Part model, mm, in its own coordinate system. Face numbers are marked on the shaded views. A direction names the side the tool comes from. Give positions to 0.01 mm unless a question says otherwise; leave off trailing zeros. Order: outer loops, then holes, each group sorted by start corner. A loop starts at its lowest first (then second) coordinate and runs counter-clockwise, first axis right, second up. Notation, with made-up numbers: M 65,37.25 L 111,37.25 A14 cw 111,62.25 Z; hole C 56,-14 d8. An arc over 180 degrees is marked long. One line per question, with ' | ' between items.
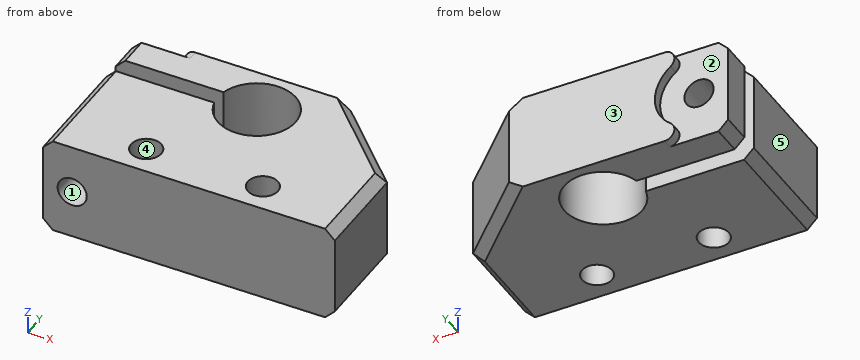
```python
from build123d import *

# Parameters (mm, degrees)
SKETCH3_W                    = 30
SKETCH3_H                    = 8
SKETCH3_R                    = 1.55
BOSS_EXTRUDE1_DEPTH          = 5
SKETCH6_R                    = 4
BOSS_EXTRUDE2_DEPTH          = 10
SKETCH8_W                    = 15
SKETCH8_H                    = 1.8
CUT_EXTRUDE_THIN1_DEPTH      = 1
CUT_EXTRUDE_THIN1_DEPTH_BACK = 11
SKETCH9_R                    = 1.5
CUT_EXTRUDE1_DEPTH           = 19
CUT_EXTRUDE2_DEPTH           = 1
CHAMFER2_SIZE                = 1


with BuildPart() as part:
    # Sketch3 → Boss-Extrude1 (new body, symmetric)
    with BuildSketch(Plane.XY):
        Rectangle(SKETCH3_W, SKETCH3_H)
        with Locations((-6, -1)):
            Circle(SKETCH3_R, mode=Mode.SUBTRACT)
        with Locations((6, -1)):
            Circle(SKETCH3_R, mode=Mode.SUBTRACT)
    extrude(amount=BOSS_EXTRUDE1_DEPTH, both=True)

    # Sketch6 → Boss-Extrude2 (add)
    with BuildSketch(Plane.XY.offset(5)):
        Polygon((-15, 4), (15, 4), (15, 6), (7, 14), (-15, 14), align=None)
        with Locations((0, 9)):
            Circle(SKETCH6_R, mode=Mode.SUBTRACT)
    extrude(amount=-BOSS_EXTRUDE2_DEPTH)

    # Sketch8 → Cut-Extrude-Thin1 (cut, two sides)
    with BuildSketch(Plane.XY.offset(5)) as cut_extrude_thin1_sk:
        with Locations((-7.5, 9)):
            Rectangle(SKETCH8_W, SKETCH8_H)
    extrude(amount=CUT_EXTRUDE_THIN1_DEPTH, mode=Mode.SUBTRACT)
    extrude(cut_extrude_thin1_sk.sketch, amount=-CUT_EXTRUDE_THIN1_DEPTH_BACK, mode=Mode.SUBTRACT)

    # Sketch9 → Cut-Extrude1 (cut, through all)
    with BuildSketch(Plane(origin=(0, 14, 0), x_dir=(1, 0, 0), z_dir=(0, 1, 0))):
        with Locations((-12, 0)):
            Circle(SKETCH9_R)
    extrude(amount=-CUT_EXTRUDE1_DEPTH, mode=Mode.SUBTRACT)

    # Sketch10 → Cut-Extrude2 (cut)
    with BuildSketch(Plane(origin=(0, 14, 0), x_dir=(1, 0, 0), z_dir=(0, 1, 0))):
        with BuildLine():
            Line((-9, 5), (-15, 5))
            Line((-15, 5), (-15, -5))
            Line((-15, -5), (-9, -5))
            ThreePointArc((-9, -5), (-9.948683298, -4.316227766), (-9.6, -3.2))
            ThreePointArc((-9.6, -3.2), (-8, 0), (-9.6, 3.2))
            ThreePointArc((-9.6, 3.2), (-9.948683298, 4.316227766), (-9, 5))
        make_face()
    extrude(amount=-CUT_EXTRUDE2_DEPTH, mode=Mode.SUBTRACT)

    # Chamfer2
    chamfer2_edges = [part.edges().sort_by_distance(p)[0] for p in [
        (11, 10, -5),
        (11, 10, 5),
        (-15, 2.05, -5),
        (-15, 2.05, 5),
        (15, 1, 5),
        (15, 1, -5),
        (-15, 11.45, -5),
        (-15, 11.45, 5),
    ]]
    chamfer(chamfer2_edges, length=CHAMFER2_SIZE)


solid = part.part
```
1. Slice it at C-C on y = -1. Give the cut face in (x, z), then the cut area to 3 significant figures.
Worked out:
outline: M -15,-4 L -14,-5 L -7.55,-5 L -7.55,5 L -14,5 L -15,4 Z; M -4.45,-5 L 4.45,-5 L 4.45,5 L -4.45,5 Z; M 7.55,-5 L 14,-5 L 15,-4 L 15,4 L 14,5 L 7.55,5 Z; hole C -12,0 d3 | area: 229 mm2
2. Slice it at A-A on z = 0. Give the cut face in (x, y).
Worked out:
outline: M -15,-4 L -13.5,-4 L -13.5,8.1 L -15,8.1 Z; M -15,9.9 L -13.5,9.9 L -13.5,13 L -15,13 Z; M -10.5,-4 L 15,-4 L 15,6 L 7,14 L -8,14 L -8,13 L -10.5,13 L -10.5,9.9 L -3.9,9.9 A4 cw long -3.9,8.1 L -10.5,8.1 Z; hole C -6,-1 d3.1; hole C 6,-1 d3.1
3. Slice it at D-D on y = 2.5. Give the cut face in (x, z), then the cut area to 3 significant figures.
Worked out:
outline: M -15,-4 L -14,-5 L 14,-5 L 15,-4 L 15,4 L 14,5 L -14,5 L -15,4 Z; hole C -12,0 d3 | area: 291 mm2
4. Slice it at B-B on x = 0. Give the cut face in (y, z).
Worked out:
outline: M -4,-5 L 5,-5 L 5,5 L -4,5 Z; M 13,-5 L 14,-5 L 14,5 L 13,5 Z
5. Mould opens along X. For the marked faces 3, 4 and 5 say: released by +X, released by -X, zero draft, split by the parting line, or undercut.
Worked out:
face 3: zero draft | face 4: undercut | face 5: released by -X
6. Drop a flat-ended pin along its axis: pin 1 (5.5 mm diameter, centred on x = -12, z = 0, fed in from +Y). Give the stop position or say it passes through.
Worked out:
pin 1: stops at y = 13
7. Tool access for the marked faces 1 and 2: list every direction of +Z, -Z, +X, -X, +Y, -Y with a clear straight run to the whole face (end or side of a thin tool).
Worked out:
face 1: +Y, -Y | face 2: -X, +Y
8. Probe L1, parallel to X at y = 6.5, z = 1.25; L2, parallel to Y at x = 6, z = -1.25; L3, parallel to Z at x = -12, y = 11.15. List the from-to ranges inside material, lowest first. Write a range as from..to.
Worked out:
L1: x = -15..-12.83, -11.17..-3.12, 3.12..14.5 | L2: y = -4..-2.55, 0.55..14 | L3: z = -5..-1.5, 1.5..5
